Autodesk Inventor part; units mm, degrees
ref_plane "YZ Plane" through (0, 0, 0) normal (1, 0, 0) x (0, 1, 0)
ref_plane "XZ Plane" through (0, 0, 0) normal (0, 1, 0) x (-1, 0, 0)
ref_plane "XY Plane" through (0, 0, 0) normal (0, 0, 1) x (1, 0, 0)
sketch "Sketch1" plane through (0, 0, 0) normal (0, 1, 0) x (-1, 0, 0)
  line L0 (-20, 20) -> (20, 20)
  line L1 (20, 20) -> (20, -20)
  line L2 (20, -20) -> (-20, -20)
  line L3 (-20, -20) -> (-20, 20)
  line L4 (-20, 20) -> (20, -20) construction
  line L5 (20, 20) -> (-20, -20) construction
  line L6 (-17, 17) -> (17, 17)
  line L7 (17, 17) -> (17, -17)
  line L8 (17, -17) -> (-17, -17)
  line L9 (-17, -17) -> (-17, 17)
  line L10 (-17, 17) -> (17, -17) construction
  line L11 (17, 17) -> (-17, -17) construction
  point P0 (0, 0)
  dimension "d0" = 40
  dimension "d1" = 40
  dimension "d2" = 34
  dimension "d3" = 34
  dimension "d4" = 3
extrude "Extrusion1" add sketch "Sketch1" along normal blind 390
sketch "Sketch2" plane through (20, 0, 20) normal (1, 0, 0) x (0, 0, -1)
  point P0 (20, 0)
properties part number "Tube 40 cm"
Geometry check sheet. Reference: the model listing, model coordinates, mm. A direction names the side the tool comes from. Round coordinates to 2 decimals unless told otherwise and drop trailing zeros. Loops run counter-clockwise (first coordinate to the right, second up) from the corner with the lowest first, then second, coordinate; pieces in that order, holes last. Notation, with made-up numbers: (45, 7.25) - (51, 7.25) arc R21 cw to (51, 25.25) - close; hole circle Ø8 at (68, 75.5). An arc over 180 degrees is marked (long way). Write item = value, one per line. Start each with the question number.
1. Mould release check, pull along Z, two halves, no side actions. Record for faces 1 (the face through (0, 192, -17)), 2 (the face through (0, 192, 20)), 3 (the face through (18, 0, 0)): released by +Z, released by -Z, zero draft, split by the parting line, or undercut.
2. Section check B-B on z = -10. Enter the section's corners in (x, y).
3. Depth check by flat-ended pin: pin 1 (2 mm diameter, centred on x = 9, z = 15, fed in from -Y). Enter the tip coordinate at first touch or a pass-through.
4. Thickness scan on line 1 (Z direction, x = -12.5, y = 210). Record the ranges inside material, lowest first.
5. Section check C-C on y = 292.5. Enter the section's corners in (x, z), then the cut area to 3 significant figures.
6. Set-up check for faces 4 (the face through (20, 192, 0)), 5 (the face through (0, 192, 17)): record each of +Z, -Z, +X, -X, +Y, -Y from which the full face is reachable in a straight line by a thin tool's end or side.
7. Section check A-A on x = 1.5. Enter the section's corners in (y, z), then the cut area to 3 significant figures.
Working result:
q1.face_1 = undercut
q1.face_2 = released by +Z
q1.face_3 = zero draft
q2.outline = (-20, 0) - (-17, 0) - (-17, 390) - (-20, 390) - close; (17, 0) - (20, 0) - (20, 390) - (17, 390) - close
q3.pin_1 = through
q4.line_1 = -20 to -17, 17 to 20
q5.outline = (-20, -20) - (20, -20) - (20, 20) - (-20, 20) - close; hole (-17, -17) - (17, -17) - (17, 17) - (-17, 17) - close
q5.area = 444 mm^2
q6.face_4 = +Z, -Z, +X, +Y, -Y
q6.face_5 = +Y, -Y
q7.outline = (0, -20) - (390, -20) - (390, -17) - (0, -17) - close; (0, 17) - (390, 17) - (390, 20) - (0, 20) - close
q7.area = 2,340 mm^2
